Could you check a few things on this drawing? It's one solid part, dimensions in mm from its lowest x, y, z. Give positions to 0.01 mm unless a question says otherwise; leave off trailing zeros. Write each loop counter-clockwise with the first axis right and the second up, starting at its lowest first coordinate (ties: lowest second). Pieces come first, ordered by that corner, then holes. Notation, with made-up numbers: M -1,52.25 L 7,52.25 A14 ccw 7,60.25 Z; hole C 9.5,87.25 d11. An arc over 180 degrees is marked long. Answer as CSV lines item,"result". Start each with the question number.
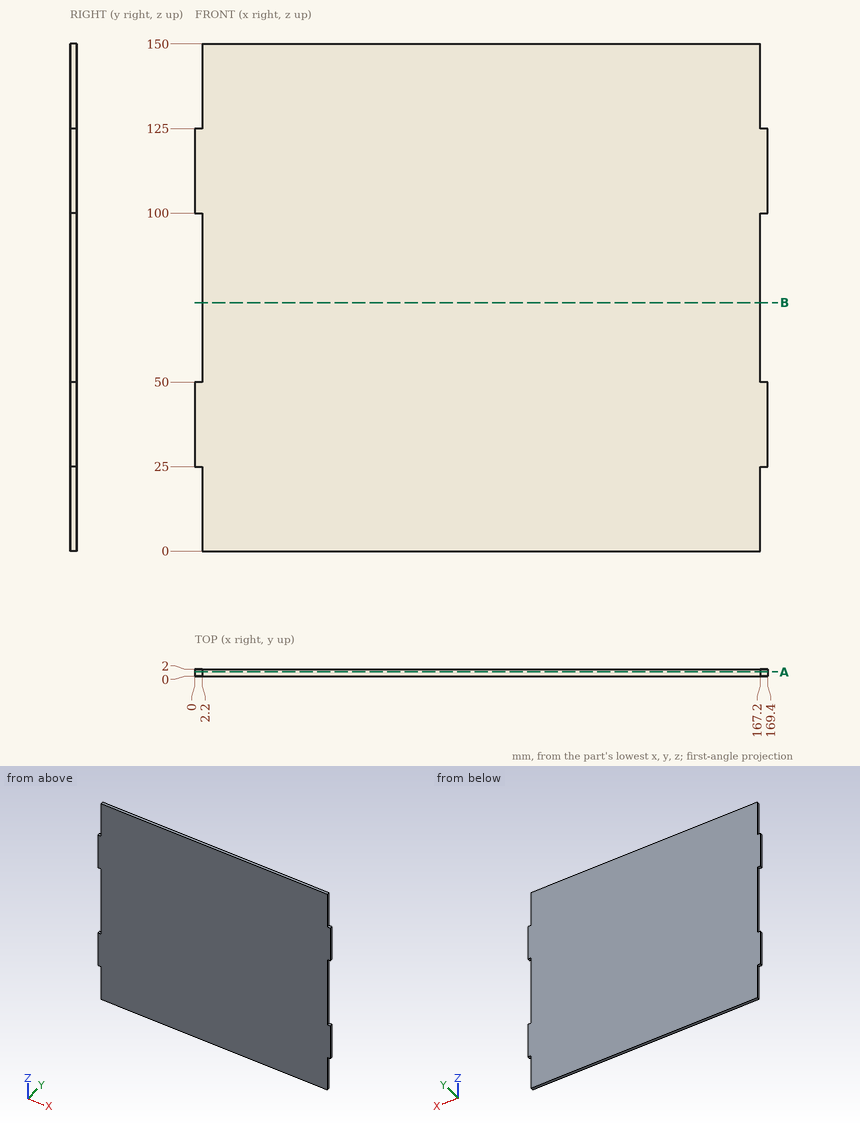
1) I want a section at A-A, the plane y = 1.25. Please give me the cut outline in (x, z).
2) I need wall thicknesses on L1, parallel to X at y = 1.3, z = 75.5. Which ranges of the line are inside material? Lowest first, please. Write a range as from..to.
3) I'm going to push flat-ended pins straight in: P1, Ø0.6, axis at x = 168.5, y = 1, coming from the -Z side; P2, Ø0.6, axis at x = 1.5, y = 0.5, coming from the +Z side; P3, Ø1, axis at y = 1.5, z = 18, coming from the +X side. Where does each tip first touch, or does it pass through?
4) I want a section at B-B, the plane z = 73.5. Please give me the cut outline in (x, y).
Values found:
1,outline,"M 0,25 L 2.2,25 L 2.2,0 L 167.2,0 L 167.2,25 L 169.4,25 L 169.4,50 L 167.2,50 L 167.2,100 L 169.4,100 L 169.4,125 L 167.2,125 L 167.2,150 L 2.2,150 L 2.2,125 L 0,125 L 0,100 L 2.2,100 L 2.2,50 L 0,50 Z"
2,L1,"x = 2.2..167.2"
3,P1,"stops at z = 25"
3,P2,"stops at z = 125"
3,P3,"stops at x = 167.2"
4,outline,"M 2.2,0 L 167.2,0 L 167.2,2 L 2.2,2 Z"
